Here's the drawing with two shaded views (mm, measured from the low corner). I have some questions. Coordinates: 2 decimals unless noted, no trailing zeros. Order: outer loops, then holes, each group sorted by start corner. A loop starts at its lowest first (then second) coordinate and runs counter-clockwise, first axis right, second up. Notation, with made-up numbers: (-40, 83) -> (-11, 83) arc R18 ccw to (-11, 118) -> close; hole circle Ø7 at (27.5, 32). An arc over 180 degrees is marked (long way). Answer as a JSON object with one key per item and string values. Group by question number.
(1) I need wall thicknesses on line 1 (Y direction, x = 134.5, z = 0.9) (1 decimal); line 2 (X direction, y = 132.5, z = 0.45); line 3 (X direction, y = 88, z = 1.85). Which ranges of each line are inside material? Lowest first, please.
(2) I want a section at C-C, the plane z = 2.2. List the corners of the cut face in (x, y) for me, plus the area to 3 significant figures.
(3) I want a section at A-A, the plane x = 100. List the corners of the cut face in (y, z) for me, plus the area to 3 significant figures.
(4) I want a section at B-B, the plane y = 150. List the corners of the cut face in (x, z) for me, plus the area to 3 significant figures.
(5) For pin 1 (6.5 mm diameter, centred on x = 33.71, y = 83.71, fed in from -Z), with a flat end and sliding along its axis, tell me the tip position at first contact or that it passes through.
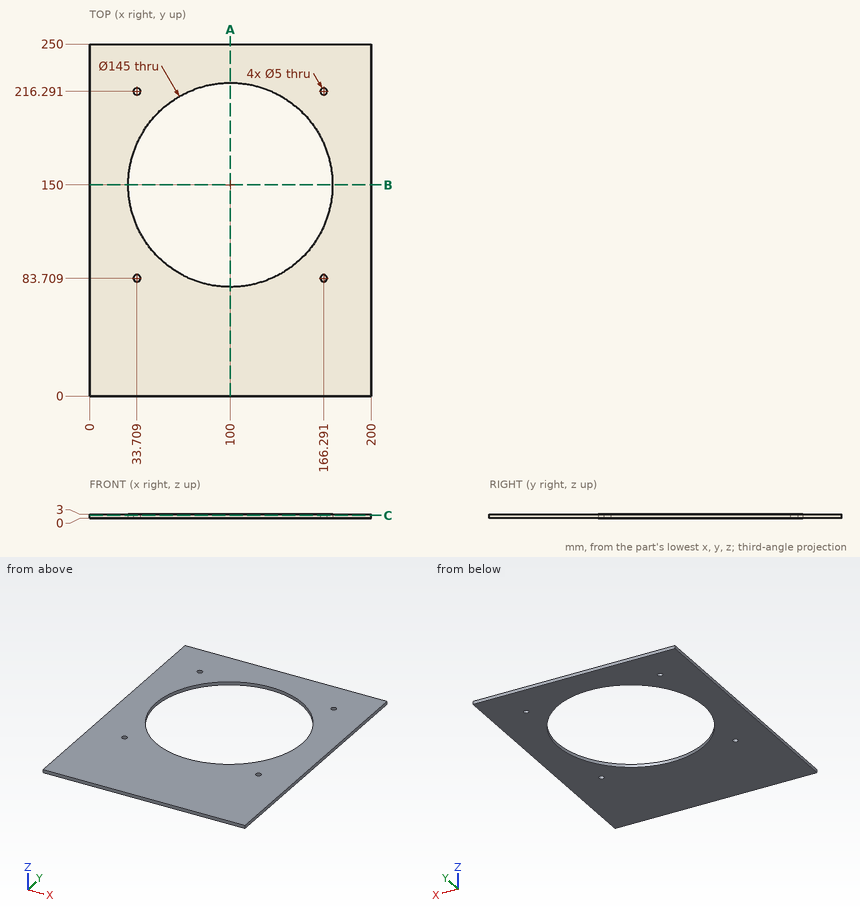
Computed values:
{
 "1": {"line 1": "y = 0 to 86.2, 213.8 to 250", "line 2": "x = 0 to 29.64, 170.36 to 200", "line 3": "x = 0 to 62.42, 137.58 to 200"},
 "2": {"outline": "(0, 0) -> (200, 0) -> (200, 250) -> (0, 250) -> close; hole circle Ø145 at (100, 150); hole circle Ø5 at (33.71, 83.71); hole circle Ø5 at (33.71, 216.29); hole circle Ø5 at (166.29, 83.71); hole circle Ø5 at (166.29, 216.29)", "area": "33,400 mm2"},
 "3": {"outline": "(0, 0) -> (77.5, 0) -> (77.5, 3) -> (0, 3) -> close; (222.5, 0) -> (250, 0) -> (250, 3) -> (222.5, 3) -> close", "area": "315 mm2"},
 "4": {"outline": "(0, 0) -> (27.5, 0) -> (27.5, 3) -> (0, 3) -> close; (172.5, 0) -> (200, 0) -> (200, 3) -> (172.5, 3) -> close", "area": "165 mm2"},
 "5": {"pin 1": "stops at z = 0"}
}
